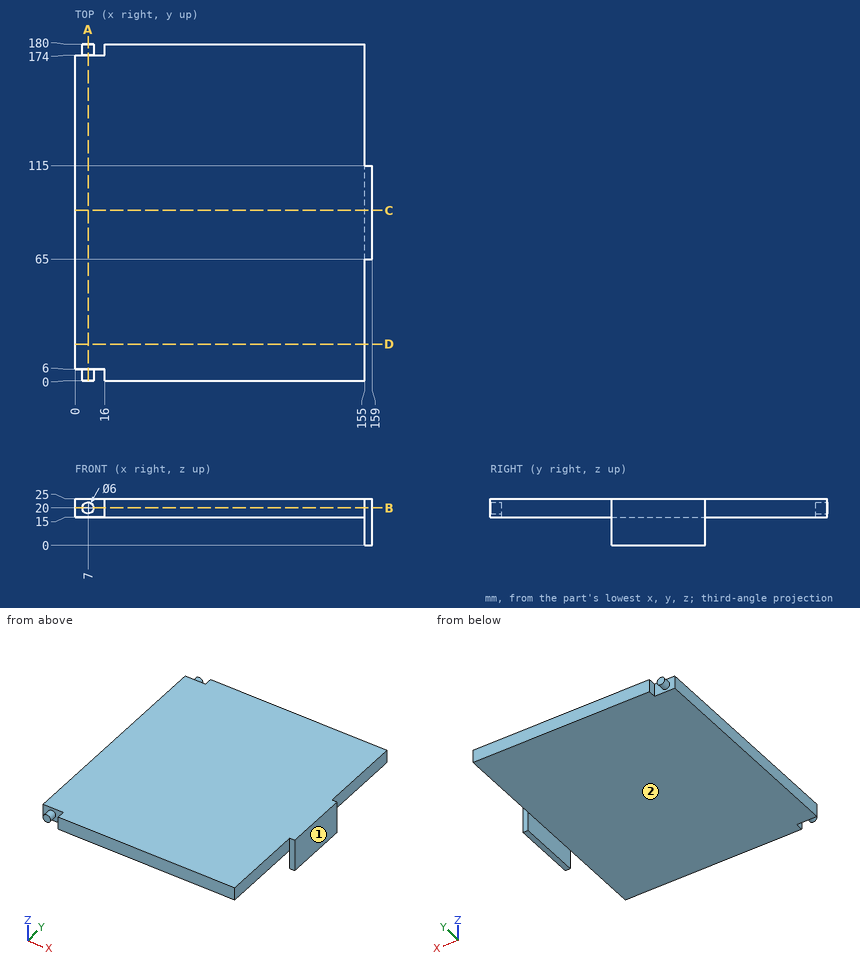
For this review, use the dimensioned drawing (mm, ordinates from the lowest corner) and the shaded views. A direction names the side the tool comes from. Give positions to 0.01 mm unless a question says otherwise; leave off trailing zeros. Loops run counter-clockwise (first coordinate to the right, second up) from the corner with the lowest first, then second, coordinate; pieces in that order, holes last.
Item 1: Take a section at C-C, the plane y = 91. State the section outline as (x, z) points, and give its area (3 significant figures).
Item 2: Tool access review of the marked faces 1 and 2: name each direction out of +Z, -Z, +X, -X, +Y, -Y from which nothing blocks a thin tool from reaching the whole face with its end or side.
Item 3: Take a section at A-A, the plane x = 7. State the section outline as (y, z) points, and give its area (3 significant figures).
Item 4: Take a section at B-B, the plane z = 20. State the section outline as (x, y) points, and give its area (3 significant figures).
Item 5: Insertion check: pin 1 (3 mm diameter, centred on y = 176.5, z = 19, fed in from -X); pin 2 (3 mm diameter, centred on y = 47, z = 19.5, fed in from +X); pin 3 (3 mm diameter, centred on x = 115.5, y = 69.5, fed in from -Z). Each pin has a flat end and moves straight along its axis. Give the tip position at first contact, or say it passes through.
Item 6: Take a section at D-D, the plane y = 19.5. State the section outline as (x, z) points, and give its area (3 significant figures).
Item 7: For line 1 along Z through (x, y) = (68, 55); line 2 along X through (y, z) = (143.5, 20.5); line 3 along X through (y, z) = (82, 14.75), list the stretches that pass through material, from the lowest coordinate up.
Calculated:
1. outline: (0, 15) - (155, 15) - (155, 0) - (159, 0) - (159, 25) - (0, 25) - close
1. area: 1,650 mm2
2. face 1: +Z, -Z, +X, +Y, -Y
2. face 2: -Z, -X, +Y, -Y
3. outline: (0, 17) - (6, 17) - (6, 15) - (174, 15) - (174, 17) - (180, 17) - (180, 23) - (174, 23) - (174, 25) - (6, 25) - (6, 23) - (0, 23) - close
3. area: 1,750 mm2
4. outline: (0, 6) - (4, 6) - (4, 0) - (10, 0) - (10, 6) - (16, 6) - (16, 0) - (155, 0) - (155, 65) - (159, 65) - (159, 115) - (155, 115) - (155, 180) - (16, 180) - (16, 174) - (10, 174) - (10, 180) - (4, 180) - (4, 174) - (0, 174) - close
4. area: 28,000 mm2
5. pin 1: stops at x = 4
5. pin 2: stops at x = 155
5. pin 3: stops at z = 15
6. outline: (0, 15) - (155, 15) - (155, 25) - (0, 25) - close
6. area: 1,550 mm2
7. line 1: z = 15 to 25
7. line 2: x = 0 to 155
7. line 3: x = 155 to 159
